```python
from build123d import *

# Parameters (mm, degrees)
SKETCH1_W           = 61
SKETCH1_H           = 61
SKETCH1_W_2         = 41
SKETCH1_H_2         = 41
BOSS_EXTRUDE1_DEPTH = 15
SKETCH2_W           = 61
SKETCH2_H           = 61
BOSS_EXTRUDE2_DEPTH = 20
SKETCH3_R           = 2.5
CUT_EXTRUDE1_DEPTH  = 90
SKETCH5_W           = 31
SKETCH5_H           = 18
CUT_EXTRUDE2_DEPTH  = 90
SKETCH6_W           = 4
SKETCH6_H           = 8
CUT_EXTRUDE3_DEPTH  = 90
SKETCH7_R           = 4.5
CUT_EXTRUDE4_DEPTH  = 5
SKETCH8_W           = 10
SKETCH8_H           = 5
CUT_EXTRUDE5_DEPTH  = 13
FILLET1_R           = 3


with BuildPart() as part:
    # Sketch1 → Boss-Extrude1 (new body)
    with BuildSketch(Plane(origin=(0, 0, 0), x_dir=(1, 0, 0), z_dir=(0, 1, 0))):
        with Locations((-20.5, 0)):
            Rectangle(SKETCH1_W, SKETCH1_H)
        with Locations((-20.5, 0)):
            Rectangle(SKETCH1_W_2, SKETCH1_H_2, mode=Mode.SUBTRACT)
    extrude(amount=BOSS_EXTRUDE1_DEPTH)

    # Sketch2 → Boss-Extrude2 (add)
    with BuildSketch(Plane(origin=(0, 15, 0), x_dir=(1, 0, 0), z_dir=(0, 1, 0))):
        with Locations((-20.5, 0)):
            Rectangle(SKETCH2_W, SKETCH2_H)
    extrude(amount=BOSS_EXTRUDE2_DEPTH)

    # Sketch3 → Cut-Extrude1 (cut)
    with BuildSketch(Plane.XY.offset(30.5)):
        with Locations((-20.5, 27.5)):
            Circle(SKETCH3_R)
        Polygon((-51, 17), (-31, 35), (-51, 35), align=None)
        Polygon((-10, 35), (10, 17), (10, 35), align=None)
    extrude(amount=-CUT_EXTRUDE1_DEPTH, mode=Mode.SUBTRACT)

    # Sketch5 → Cut-Extrude2 (cut)
    with BuildSketch(Plane(origin=(10, 0, 0), x_dir=(0, 0, -1), z_dir=(1, 0, 0))):
        with Locations((0, 26)):
            Rectangle(SKETCH5_W, SKETCH5_H)
    extrude(amount=-CUT_EXTRUDE2_DEPTH, mode=Mode.SUBTRACT)

    # Sketch6 → Cut-Extrude3 (cut)
    with BuildSketch(Plane(origin=(0, 17, 0), x_dir=(1, 0, 0), z_dir=(0, 1, 0))):
        with Locations((-49, 0)):
            Rectangle(SKETCH6_W, SKETCH6_H)
        with Locations((8, 0)):
            Rectangle(SKETCH6_W, SKETCH6_H)
    extrude(amount=-CUT_EXTRUDE3_DEPTH, mode=Mode.SUBTRACT)

    # Sketch7 → Cut-Extrude4 (cut)
    with BuildSketch(Plane.XY.offset(30.5)):
        with Locations((-20.5, 27.5)):
            Circle(SKETCH7_R)
    extrude(amount=-CUT_EXTRUDE4_DEPTH, mode=Mode.SUBTRACT)

    # Sketch8 → Cut-Extrude5 (cut)
    with BuildSketch(Plane(origin=(0, 35, 0), x_dir=(1, 0, 0), z_dir=(0, 1, 0))):
        with Locations((-20.5, 22)):
            Rectangle(SKETCH8_W, SKETCH8_H)
    extrude(amount=-CUT_EXTRUDE5_DEPTH, mode=Mode.SUBTRACT)

    # Fillet1
    fillet1_edges = [part.edges().sort_by_distance(p)[0] for p in [
        (6, 17, 0),
        (-47, 17, 0),
    ]]
    fillet(fillet1_edges, radius=FILLET1_R)


solid = part.part
```
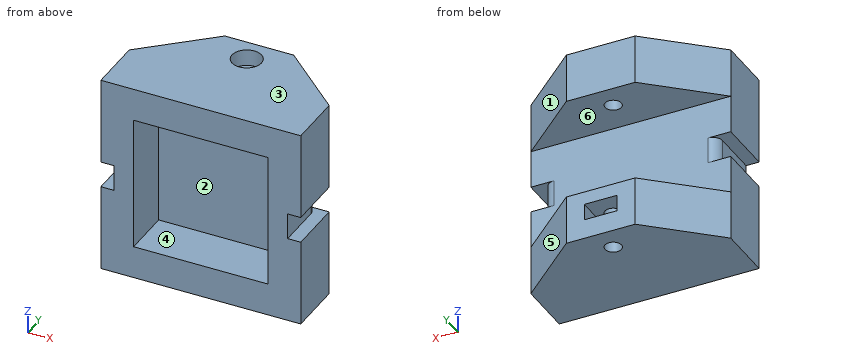
Design review of the part built by this model. Coordinates are the model's own, in mm. Face numbers are marked on the shaded views. A direction names the side the tool comes from. Coordinates: 2 decimals unless noted, no trailing zeros. Order: outer loops, then holes, each group sorted by start corner. A loop starts at its lowest first (then second) coordinate and runs counter-clockwise, first axis right, second up. Notation, with made-up numbers: (53, 47) -> (86, 47) arc R25 cw to (86, 71) -> close; hole circle Ø7 at (25, 37.25). An arc over 180 degrees is marked (long way). One line per item, written item: value. Start each with the question number.
Q1. For probe 1 along Y at (x, z) = (-20.5, 20.25); probe 2 along Z at (x, y) = (-26.5, 9); probe 3 along Y at (x, z) = (-20.5, 23.5), list the stretches that pass through material, from the lowest coordinate up.
Q2. Take a section at A-A, the plane x = -20.5. Give the number of separate pieces and of enclosed holes in the cut face, then the cut area to 3 significant figures.
Q3. Insertion check: pin 1 Ø4.5 at (x, y) = (-20.5, 27.5) entering from +Z; pin 2 Ø1.5 at (y, z) = (29.5, -23) entering from -X; pin 3 Ø7.5 at (y, z) = (4, 0) entering from +X; pin 4 Ø5 at (x, z) = (-17, 5.5) entering from +Y. Each pin has a flat end and moves straight along its axis. Give the tip position at first contact, or say it passes through.
Q4. Take a section at B-B, the plane y = 6. State the section outline as (x, z) points.
Q5. Mouldability with a two-part tool opening along Z and no side actions: class the marked faces 1, 2 and 3 as pulls with the +Z half, pulls with the -Z half, needs draft (parallel to the pull), parting line crosses it, or undercut.
Q6. Take a section at D-D, the plane y = 27.5. State the section outline as (x, z) points, then the cut area to 3 significant figures.
Q7. Tool access review of the marked faces 4, 5 and 6: name each direction out of +Z, -Z, +X, -X, +Y, -Y from which nothing blocks a thin tool from reaching the whole face with its end or side.
Q8. Take a section at C-C, the plane z = 2. State the section outline as (x, y) points.
Values follow:
1. probe 1: y = 15 to 25, 30 to 35
1. probe 2: z = -30.5 to -20.5, 20.5 to 30.5
1. probe 3: y = 0 to 25, 30 to 35
2. separate pieces: 4
2. enclosed holes: 0
2. area: 752 mm2
3. pin 1: passes through
3. pin 2: stops at x = -37.94
3. pin 3: stops at x = 6
3. pin 4: stops at y = 17
4. outline: (-51, -30.5) -> (10, -30.5) -> (10, -4) -> (6, -4) -> (6, 4) -> (10, 4) -> (10, 30.5) -> (-51, 30.5) -> (-51, 4) -> (-47, 4) -> (-47, -4) -> (-51, -4) -> close; hole (-41, -20.5) -> (0, -20.5) -> (0, 20.5) -> (-41, 20.5) -> close
5. face 1: needs draft
5. face 2: undercut
5. face 3: pulls with the +Z half
6. outline: (-39.33, -30.5) -> (-23, -30.5) -> (-23, -24.5) -> (-25.5, -24.5) -> (-25.5, -19.5) -> (-23, -19.5) -> (-23, -15.5) -> (-39.33, -15.5) -> close; (-39.33, 15.5) -> (-23, 15.5) -> (-23, 25.5) -> (-25, 25.5) -> (-25, 30.5) -> (-39.33, 30.5) -> close; (-18, -30.5) -> (-1.67, -30.5) -> (-1.67, -15.5) -> (-18, -15.5) -> (-18, -19.5) -> (-15.5, -19.5) -> (-15.5, -24.5) -> (-18, -24.5) -> close; (-18, 15.5) -> (-1.67, 15.5) -> (-1.67, 30.5) -> (-16, 30.5) -> (-16, 25.5) -> (-18, 25.5) -> close
6. area: 935 mm2
7. face 4: -Y
7. face 5: +Z, -Z, +X, +Y
7. face 6: +X, -X, +Y
8. outline: (-47, 0) -> (-41, 0) -> (-41, 15) -> (0, 15) -> (0, 0) -> (6, 0) -> (6, 14) arc R3 ccw to (3, 17) -> (-44, 17) arc R3 ccw to (-47, 14) -> close
